The listing builds one solid part. Answer for the finished solid, in the listing's coordinates (mm). Face numbers are marked on the shaded views. A direction names the side the tool comes from. Coordinates: 2 decimals unless noted, no trailing zeros. Order: outer loops, then holes, each group sorted by start corner. A loop starts at its lowest first (then second) coordinate and runs counter-clockwise, first axis right, second up. Notation, with made-up numbers: (-6.5, -40) -> (26.5, -40) arc R23 ccw to (26.5, -1) -> close; hole circle Ø7 at (39.5, 2). An arc over 180 degrees is marked (long way). Answer in a Markdown table with one row per item.
```python
from build123d import *

# Parameters (mm, degrees)
SKETCH_1_R               = 21.875
EXTRUDE_1_DEPTH          = 15
PATTERN_CIRCULAR_1_COUNT = 20
SKETCH_3_R               = 15
CUT_EXTRUDE_1_DEPTH      = 44.09328544
CUT_EXTRUDE_4_DEPTH      = 35.380681349
CUT_EXTRUDE_4_DEPTH_BACK = 35.380681349
SKETCH_6_W               = 3
SKETCH_6_H               = 17
SKETCH_7_R               = 26.875
SKETCH_7_R_2             = 21.875
EXTRUDE_2_DEPTH          = 5


with BuildPart() as part:
    # Sketch 1 → Extrude 1 (new, symmetric)
    with BuildSketch(Plane.XY):
        Circle(SKETCH_1_R)
    extrude(amount=EXTRUDE_1_DEPTH, both=True)


with BuildPart() as pattern_circular_1_1:
    # Pattern Circular 1: pattern copy
    add(part.part.rotate(Axis((0, 0, 15), (0, 0, 1)), 1 * 360 / PATTERN_CIRCULAR_1_COUNT))


with BuildPart() as pattern_circular_1_2:
    # Pattern Circular 1: pattern copy
    add(part.part.rotate(Axis((0, 0, 15), (0, 0, 1)), 2 * 360 / PATTERN_CIRCULAR_1_COUNT))


with BuildPart() as pattern_circular_1_3:
    # Pattern Circular 1: pattern copy
    add(part.part.rotate(Axis((0, 0, 15), (0, 0, 1)), 3 * 360 / PATTERN_CIRCULAR_1_COUNT))


with BuildPart() as pattern_circular_1_4:
    # Pattern Circular 1: pattern copy
    add(part.part.rotate(Axis((0, 0, 15), (0, 0, 1)), 4 * 360 / PATTERN_CIRCULAR_1_COUNT))


with BuildPart() as pattern_circular_1_5:
    # Pattern Circular 1: pattern copy
    add(part.part.rotate(Axis((0, 0, 15), (0, 0, 1)), 5 * 360 / PATTERN_CIRCULAR_1_COUNT))


with BuildPart() as pattern_circular_1_6:
    # Pattern Circular 1: pattern copy
    add(part.part.rotate(Axis((0, 0, 15), (0, 0, 1)), 6 * 360 / PATTERN_CIRCULAR_1_COUNT))


with BuildPart() as pattern_circular_1_7:
    # Pattern Circular 1: pattern copy
    add(part.part.rotate(Axis((0, 0, 15), (0, 0, 1)), 7 * 360 / PATTERN_CIRCULAR_1_COUNT))


with BuildPart() as pattern_circular_1_8:
    # Pattern Circular 1: pattern copy
    add(part.part.rotate(Axis((0, 0, 15), (0, 0, 1)), 8 * 360 / PATTERN_CIRCULAR_1_COUNT))


with BuildPart() as pattern_circular_1_9:
    # Pattern Circular 1: pattern copy
    add(part.part.rotate(Axis((0, 0, 15), (0, 0, 1)), 9 * 360 / PATTERN_CIRCULAR_1_COUNT))


with BuildPart() as pattern_circular_1_10:
    # Pattern Circular 1: pattern copy
    add(part.part.rotate(Axis((0, 0, 15), (0, 0, 1)), 10 * 360 / PATTERN_CIRCULAR_1_COUNT))


with BuildPart() as pattern_circular_1_11:
    # Pattern Circular 1: pattern copy
    add(part.part.rotate(Axis((0, 0, 15), (0, 0, 1)), 11 * 360 / PATTERN_CIRCULAR_1_COUNT))


with BuildPart() as pattern_circular_1_12:
    # Pattern Circular 1: pattern copy
    add(part.part.rotate(Axis((0, 0, 15), (0, 0, 1)), 12 * 360 / PATTERN_CIRCULAR_1_COUNT))


with BuildPart() as pattern_circular_1_13:
    # Pattern Circular 1: pattern copy
    add(part.part.rotate(Axis((0, 0, 15), (0, 0, 1)), 13 * 360 / PATTERN_CIRCULAR_1_COUNT))


with BuildPart() as pattern_circular_1_14:
    # Pattern Circular 1: pattern copy
    add(part.part.rotate(Axis((0, 0, 15), (0, 0, 1)), 14 * 360 / PATTERN_CIRCULAR_1_COUNT))


with BuildPart() as pattern_circular_1_15:
    # Pattern Circular 1: pattern copy
    add(part.part.rotate(Axis((0, 0, 15), (0, 0, 1)), 15 * 360 / PATTERN_CIRCULAR_1_COUNT))


with BuildPart() as pattern_circular_1_16:
    # Pattern Circular 1: pattern copy
    add(part.part.rotate(Axis((0, 0, 15), (0, 0, 1)), 16 * 360 / PATTERN_CIRCULAR_1_COUNT))


with BuildPart() as pattern_circular_1_17:
    # Pattern Circular 1: pattern copy
    add(part.part.rotate(Axis((0, 0, 15), (0, 0, 1)), 17 * 360 / PATTERN_CIRCULAR_1_COUNT))


with BuildPart() as pattern_circular_1_18:
    # Pattern Circular 1: pattern copy
    add(part.part.rotate(Axis((0, 0, 15), (0, 0, 1)), 18 * 360 / PATTERN_CIRCULAR_1_COUNT))


with BuildPart() as pattern_circular_1_19:
    # Pattern Circular 1: pattern copy
    add(part.part.rotate(Axis((0, 0, 15), (0, 0, 1)), 19 * 360 / PATTERN_CIRCULAR_1_COUNT))


with BuildPart() as cut_extrude_1_tool:
    # Sketch 3 → Cut-Extrude 1 (new, through all)
    with BuildSketch(Plane.XY.offset(15)):
        Circle(SKETCH_3_R)
    extrude(amount=-CUT_EXTRUDE_1_DEPTH)


with BuildPart() as part_1:
    add(part.part)

    # Cut-Extrude 1: cut by cut_extrude_1_tool
    add(cut_extrude_1_tool.part, mode=Mode.SUBTRACT)


with BuildPart() as pattern_circular_1_1_1:
    add(pattern_circular_1_1.part)

    # Cut-Extrude 1: cut by cut_extrude_1_tool
    add(cut_extrude_1_tool.part, mode=Mode.SUBTRACT)


with BuildPart() as pattern_circular_1_2_1:
    add(pattern_circular_1_2.part)

    # Cut-Extrude 1: cut by cut_extrude_1_tool
    add(cut_extrude_1_tool.part, mode=Mode.SUBTRACT)


with BuildPart() as pattern_circular_1_3_1:
    add(pattern_circular_1_3.part)

    # Cut-Extrude 1: cut by cut_extrude_1_tool
    add(cut_extrude_1_tool.part, mode=Mode.SUBTRACT)


with BuildPart() as pattern_circular_1_4_1:
    add(pattern_circular_1_4.part)

    # Cut-Extrude 1: cut by cut_extrude_1_tool
    add(cut_extrude_1_tool.part, mode=Mode.SUBTRACT)


with BuildPart() as pattern_circular_1_5_1:
    add(pattern_circular_1_5.part)

    # Cut-Extrude 1: cut by cut_extrude_1_tool
    add(cut_extrude_1_tool.part, mode=Mode.SUBTRACT)


with BuildPart() as pattern_circular_1_6_1:
    add(pattern_circular_1_6.part)

    # Cut-Extrude 1: cut by cut_extrude_1_tool
    add(cut_extrude_1_tool.part, mode=Mode.SUBTRACT)


with BuildPart() as pattern_circular_1_7_1:
    add(pattern_circular_1_7.part)

    # Cut-Extrude 1: cut by cut_extrude_1_tool
    add(cut_extrude_1_tool.part, mode=Mode.SUBTRACT)


with BuildPart() as pattern_circular_1_8_1:
    add(pattern_circular_1_8.part)

    # Cut-Extrude 1: cut by cut_extrude_1_tool
    add(cut_extrude_1_tool.part, mode=Mode.SUBTRACT)


with BuildPart() as pattern_circular_1_9_1:
    add(pattern_circular_1_9.part)

    # Cut-Extrude 1: cut by cut_extrude_1_tool
    add(cut_extrude_1_tool.part, mode=Mode.SUBTRACT)


with BuildPart() as pattern_circular_1_10_1:
    add(pattern_circular_1_10.part)

    # Cut-Extrude 1: cut by cut_extrude_1_tool
    add(cut_extrude_1_tool.part, mode=Mode.SUBTRACT)


with BuildPart() as pattern_circular_1_11_1:
    add(pattern_circular_1_11.part)

    # Cut-Extrude 1: cut by cut_extrude_1_tool
    add(cut_extrude_1_tool.part, mode=Mode.SUBTRACT)


with BuildPart() as pattern_circular_1_12_1:
    add(pattern_circular_1_12.part)

    # Cut-Extrude 1: cut by cut_extrude_1_tool
    add(cut_extrude_1_tool.part, mode=Mode.SUBTRACT)


with BuildPart() as pattern_circular_1_13_1:
    add(pattern_circular_1_13.part)

    # Cut-Extrude 1: cut by cut_extrude_1_tool
    add(cut_extrude_1_tool.part, mode=Mode.SUBTRACT)


with BuildPart() as pattern_circular_1_14_1:
    add(pattern_circular_1_14.part)

    # Cut-Extrude 1: cut by cut_extrude_1_tool
    add(cut_extrude_1_tool.part, mode=Mode.SUBTRACT)


with BuildPart() as pattern_circular_1_15_1:
    add(pattern_circular_1_15.part)

    # Cut-Extrude 1: cut by cut_extrude_1_tool
    add(cut_extrude_1_tool.part, mode=Mode.SUBTRACT)


with BuildPart() as pattern_circular_1_16_1:
    add(pattern_circular_1_16.part)

    # Cut-Extrude 1: cut by cut_extrude_1_tool
    add(cut_extrude_1_tool.part, mode=Mode.SUBTRACT)


with BuildPart() as pattern_circular_1_17_1:
    add(pattern_circular_1_17.part)

    # Cut-Extrude 1: cut by cut_extrude_1_tool
    add(cut_extrude_1_tool.part, mode=Mode.SUBTRACT)


with BuildPart() as pattern_circular_1_18_1:
    add(pattern_circular_1_18.part)

    # Cut-Extrude 1: cut by cut_extrude_1_tool
    add(cut_extrude_1_tool.part, mode=Mode.SUBTRACT)


with BuildPart() as pattern_circular_1_19_1:
    add(pattern_circular_1_19.part)

    # Cut-Extrude 1: cut by cut_extrude_1_tool
    add(cut_extrude_1_tool.part, mode=Mode.SUBTRACT)


with BuildPart() as cut_extrude_4_tool:
    # Sketch 6 → Cut-Extrude 4 (new, two sides: drawn at the far end of the back side and taken through both)
    with BuildSketch(Plane.XY.offset(-CUT_EXTRUDE_4_DEPTH_BACK)):
        with Locations((0, 8.5)):
            Rectangle(SKETCH_6_W, SKETCH_6_H)
    extrude(amount=CUT_EXTRUDE_4_DEPTH + CUT_EXTRUDE_4_DEPTH_BACK)


with BuildPart() as part_2:
    add(part_1.part)

    # Cut-Extrude 4: cut by cut_extrude_4_tool
    add(cut_extrude_4_tool.part, mode=Mode.SUBTRACT)



with BuildPart() as pattern_circular_1_1_2:
    add(pattern_circular_1_1_1.part)

    # Cut-Extrude 4: cut by cut_extrude_4_tool
    add(cut_extrude_4_tool.part, mode=Mode.SUBTRACT)


with BuildPart() as pattern_circular_1_2_2:
    add(pattern_circular_1_2_1.part)

    # Cut-Extrude 4: cut by cut_extrude_4_tool
    add(cut_extrude_4_tool.part, mode=Mode.SUBTRACT)


with BuildPart() as pattern_circular_1_3_2:
    add(pattern_circular_1_3_1.part)

    # Cut-Extrude 4: cut by cut_extrude_4_tool
    add(cut_extrude_4_tool.part, mode=Mode.SUBTRACT)


with BuildPart() as pattern_circular_1_4_2:
    add(pattern_circular_1_4_1.part)

    # Cut-Extrude 4: cut by cut_extrude_4_tool
    add(cut_extrude_4_tool.part, mode=Mode.SUBTRACT)


with BuildPart() as pattern_circular_1_5_2:
    add(pattern_circular_1_5_1.part)

    # Cut-Extrude 4: cut by cut_extrude_4_tool
    add(cut_extrude_4_tool.part, mode=Mode.SUBTRACT)


with BuildPart() as pattern_circular_1_6_2:
    add(pattern_circular_1_6_1.part)

    # Cut-Extrude 4: cut by cut_extrude_4_tool
    add(cut_extrude_4_tool.part, mode=Mode.SUBTRACT)


with BuildPart() as pattern_circular_1_7_2:
    add(pattern_circular_1_7_1.part)

    # Cut-Extrude 4: cut by cut_extrude_4_tool
    add(cut_extrude_4_tool.part, mode=Mode.SUBTRACT)


with BuildPart() as pattern_circular_1_8_2:
    add(pattern_circular_1_8_1.part)

    # Cut-Extrude 4: cut by cut_extrude_4_tool
    add(cut_extrude_4_tool.part, mode=Mode.SUBTRACT)


with BuildPart() as pattern_circular_1_9_2:
    add(pattern_circular_1_9_1.part)

    # Cut-Extrude 4: cut by cut_extrude_4_tool
    add(cut_extrude_4_tool.part, mode=Mode.SUBTRACT)


with BuildPart() as pattern_circular_1_10_2:
    add(pattern_circular_1_10_1.part)

    # Cut-Extrude 4: cut by cut_extrude_4_tool
    add(cut_extrude_4_tool.part, mode=Mode.SUBTRACT)


with BuildPart() as pattern_circular_1_11_2:
    add(pattern_circular_1_11_1.part)

    # Cut-Extrude 4: cut by cut_extrude_4_tool
    add(cut_extrude_4_tool.part, mode=Mode.SUBTRACT)


with BuildPart() as pattern_circular_1_12_2:
    add(pattern_circular_1_12_1.part)

    # Cut-Extrude 4: cut by cut_extrude_4_tool
    add(cut_extrude_4_tool.part, mode=Mode.SUBTRACT)


with BuildPart() as pattern_circular_1_13_2:
    add(pattern_circular_1_13_1.part)

    # Cut-Extrude 4: cut by cut_extrude_4_tool
    add(cut_extrude_4_tool.part, mode=Mode.SUBTRACT)


with BuildPart() as pattern_circular_1_14_2:
    add(pattern_circular_1_14_1.part)

    # Cut-Extrude 4: cut by cut_extrude_4_tool
    add(cut_extrude_4_tool.part, mode=Mode.SUBTRACT)


with BuildPart() as pattern_circular_1_15_2:
    add(pattern_circular_1_15_1.part)

    # Cut-Extrude 4: cut by cut_extrude_4_tool
    add(cut_extrude_4_tool.part, mode=Mode.SUBTRACT)


with BuildPart() as pattern_circular_1_16_2:
    add(pattern_circular_1_16_1.part)

    # Cut-Extrude 4: cut by cut_extrude_4_tool
    add(cut_extrude_4_tool.part, mode=Mode.SUBTRACT)


with BuildPart() as pattern_circular_1_17_2:
    add(pattern_circular_1_17_1.part)

    # Cut-Extrude 4: cut by cut_extrude_4_tool
    add(cut_extrude_4_tool.part, mode=Mode.SUBTRACT)


with BuildPart() as pattern_circular_1_18_2:
    add(pattern_circular_1_18_1.part)

    # Cut-Extrude 4: cut by cut_extrude_4_tool
    add(cut_extrude_4_tool.part, mode=Mode.SUBTRACT)


with BuildPart() as pattern_circular_1_19_2:
    add(pattern_circular_1_19_1.part)

    # Cut-Extrude 4: cut by cut_extrude_4_tool
    add(cut_extrude_4_tool.part, mode=Mode.SUBTRACT)


with BuildPart() as part_3:
    add(part_2.part)

    add(pattern_circular_1_1_2.part)  # Extrude 2 merges Pattern Circular 1_1

    add(pattern_circular_1_2_2.part)  # Extrude 2 merges Pattern Circular 1_2

    add(pattern_circular_1_3_2.part)  # Extrude 2 merges Pattern Circular 1_3

    add(pattern_circular_1_4_2.part)  # Extrude 2 merges Pattern Circular 1_4

    add(pattern_circular_1_5_2.part)  # Extrude 2 merges Pattern Circular 1_5

    add(pattern_circular_1_6_2.part)  # Extrude 2 merges Pattern Circular 1_6

    add(pattern_circular_1_7_2.part)  # Extrude 2 merges Pattern Circular 1_7

    add(pattern_circular_1_8_2.part)  # Extrude 2 merges Pattern Circular 1_8

    add(pattern_circular_1_9_2.part)  # Extrude 2 merges Pattern Circular 1_9

    add(pattern_circular_1_10_2.part)  # Extrude 2 merges Pattern Circular 1_10

    add(pattern_circular_1_11_2.part)  # Extrude 2 merges Pattern Circular 1_11

    add(pattern_circular_1_12_2.part)  # Extrude 2 merges Pattern Circular 1_12

    add(pattern_circular_1_13_2.part)  # Extrude 2 merges Pattern Circular 1_13

    add(pattern_circular_1_14_2.part)  # Extrude 2 merges Pattern Circular 1_14

    add(pattern_circular_1_15_2.part)  # Extrude 2 merges Pattern Circular 1_15

    add(pattern_circular_1_16_2.part)  # Extrude 2 merges Pattern Circular 1_16

    add(pattern_circular_1_17_2.part)  # Extrude 2 merges Pattern Circular 1_17

    add(pattern_circular_1_18_2.part)  # Extrude 2 merges Pattern Circular 1_18

    add(pattern_circular_1_19_2.part)  # Extrude 2 merges Pattern Circular 1_19
    # Sketch 7 → Extrude 2 (add)
    with BuildSketch(Plane.XY.offset(15)):
        Circle(SKETCH_7_R)
        Circle(SKETCH_7_R_2, mode=Mode.SUBTRACT)
    extrude_2 = extrude(amount=-EXTRUDE_2_DEPTH)

    # Mirror 1: Extrude 2 across plane
    add(extrude_2.mirror(Plane.XY))


solid = part_3.part
```
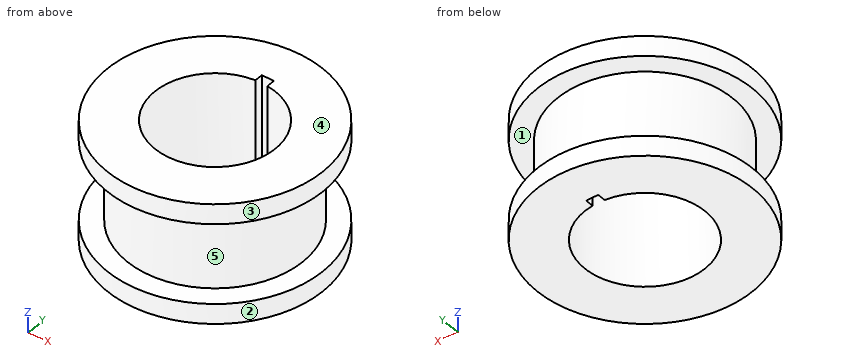
(1) Flat-ended cylindrical pins translate along their axes: pin 1 (8 mm diameter, centred on x = 12.5, z = 9.5, fed in from -Y); pin 2 (2 mm diameter, centred on x = 3.5, z = 3.5, fed in from +Y); pin 3 (10 mm diameter, centred on x = 4.5, y = -14, fed in from -Z); pin 4 (1.7 mm diameter, centred on y = 16, z = 7.5, fed in from -X). Find the tip coordinate at first contact, or state that the pin passes through.
Check values:
| item | result |
|---|---|
| pin 1 | y = -25.48 |
| pin 2 | y = 21.73 |
| pin 3 | z = -15 |
| pin 4 | x = -15.78 |
(2) Which of the six approach directions +Z, -Z, +X, -X, +Y, -Y give full straight-line access (tool end or side, diameter ignored) to the marked faces 1 and 2?
Check values:
| item | result |
|---|---|
| face 1 | none |
| face 2 | +Z, -Z |
(3) A cutting plane is placed at B-B, the plane y = 0. Determine the outline of the cut face in (x, z) (3 decimals), then the cut area to 4 significant figures.
Check values:
| item | result |
|---|---|
| outline | (-26.875, -15) -> (-15, -15) -> (-15, 15) -> (-26.875, 15) -> (-26.875, 10) -> (-21.875, 10) -> (-21.875, -10) -> (-26.875, -10) -> close; (15, -15) -> (26.875, -15) -> (26.875, -10) -> (21.875, -10) -> (21.875, 10) -> (26.875, 10) -> (26.875, 15) -> (15, 15) -> close |
| area | 512.5 mm² |
(4) A cutting plane is placed at C-C, the plane z = 0.5. Determine the outline of the cut face in (x, y) (3 decimals).
Check values:
| item | result |
|---|---|
| outline | circle Ø43.75 at (0, 0); hole (-1.5, 14.925) arc R15 ccw (long way) to (1.5, 14.925) -> (1.5, 17) -> (-1.5, 17) -> close |
(5) Find the intervals of material crossed by line 1 along Y through (x, z) = (0, -0.5) (3 decimals); line 2 along Z through (x, y) = (1, 24.5); line 3 along Y through (x, z) = (13, 7.75), in increasing order. Write a range as from..to.
Check values:
| item | result |
|---|---|
| line 1 | -21.875..-15, 17..21.875 |
| line 2 | -15..-10, 10..15 |
| line 3 | -17.59..-7.48, 7.48..17.59 |
(6) A cutting plane is placed at A-A, the plane x = 0. Determine the outline of the cut face in (y, z) (3 decimals), then the cut area to 4 significant figures.
Check values:
| item | result |
|---|---|
| outline | (-26.875, -15) -> (-15, -15) -> (-15, 15) -> (-26.875, 15) -> (-26.875, 10) -> (-21.875, 10) -> (-21.875, -10) -> (-26.875, -10) -> close; (17, -15) -> (26.875, -15) -> (26.875, -10) -> (21.875, -10) -> (21.875, 10) -> (26.875, 10) -> (26.875, 15) -> (17, 15) -> close |
| area | 452.5 mm² |
(7) A cutting plane is placed at D-D, the plane z = -11.25. Determine the outline of the cut face in (x, y) (3 decimals), then the cut area to 3 significant figures.
Check values:
| item | result |
|---|---|
| outline | circle Ø53.75 at (0, 0); hole (-1.5, 14.925) arc R15 ccw (long way) to (1.5, 14.925) -> (1.5, 17) -> (-1.5, 17) -> close |
| area | 1,560 mm² |
(8) For a pull along Z with two mould halves and no side action, classify the marked faces 3, 4 and 5 as released by +Z, released by -Z, zero draft, split by the parting line, or undercut.
Check values:
| item | result |
|---|---|
| face 3 | zero draft |
| face 4 | released by +Z |
| face 5 | undercut |
